Can you work these out from the model? Positions are in its coordinate system, mm. Face numbers are marked on the shaded views. Coordinates: 2 decimals unless noted, no trailing zeros. Loops run counter-clockwise (first coordinate to the right, second up) from the corner with the lowest first, then second, coordinate; pieces in that order, holes last.
```python
from build123d import *

# Parameters (mm, degrees)
F1_DEPTH  = 8
F3_DEPTH  = 50
F4_R      = 5
F5_DEPTH  = 9
F7_DEPTH  = 8
F9_DEPTH  = 25
F11_DEPTH = 65
F12_DEPTH = 1
F13_R     = 5
F14_R     = 2
F15_R     = 2


with BuildPart() as f1:
    # F0 (on Top) → F1 (new body)
    with BuildSketch(Plane.XY):
        Polygon((-15, 0), (0, 0), (10, 0), (10, 15), (10, 25), (5, 25), (5, 17), (-5, 17), (-13, 17), (-13, 25), (-20, 25), (-20, 0), align=None)
        with BuildLine():
            Line((10, 0), (0, 0))
            Line((0, 0), (-15, 0))
            ThreePointArc((-15, 0), (-4.7480671489, -26.7494728588), (0, -55))
            Line((0, -55), (10, -55))
            Line((10, -55), (10, 0))
        make_face()
        with BuildLine():
            ThreePointArc((16.1671913498, -8.6829612821), (13.2107261045, -4.2511845243), (10, 0))
            Line((10, 0), (10, -55))
            Line((10, -55), (30, -55))
            ThreePointArc((30, -55), (26.2150971911, -30.9062424985), (16.1671913498, -8.6829612821))
        make_face()
    extrude(amount=F1_DEPTH)

    # F2 (on face) → F3 (cut)
    with BuildSketch(Plane.YZ.offset(10)):
        with BuildLine():
            Line((22, 4), (24.5, 4))
            ThreePointArc((24.5, 4), (22, 6.5), (19.5, 4))
            Line((19.5, 4), (22, 4))
        make_face()
        with BuildLine():
            ThreePointArc((19.5, 4), (22, 1.5), (24.5, 4))
            Line((24.5, 4), (22, 4))
            Line((22, 4), (19.5, 4))
        make_face()
    extrude(amount=-F3_DEPTH, mode=Mode.SUBTRACT)

    # F4 (on face) → F5 (join)
    with BuildSketch(Plane(origin=(0, 0, 0), x_dir=(1, 0, 0), z_dir=(0, 0, -1))):
        with Locations((5, 0)):
            Circle(F4_R)
    extrude(amount=-F5_DEPTH)

    # F6 (on face) → F7 (join)
    with BuildSketch(Plane.XY.offset(9)):
        with BuildLine():
            ThreePointArc((1.05, 0), (5, -3.95), (8.95, 0))
            Line((8.95, 0), (1.05, 0))
        make_face()
        with BuildLine():
            Line((1.05, 0), (8.95, 0))
            ThreePointArc((8.95, 0), (5, 3.95), (1.05, 0))
        make_face()
    extrude(amount=F7_DEPTH)

    # F8 (on face) → F9 (cut)
    with BuildSketch(Plane.XY.offset(17)):
        with BuildLine():
            Line((2.5, 0), (7.5, 0))
            ThreePointArc((7.5, 0), (5, 2.5), (2.5, 0))
        make_face()
        with BuildLine():
            ThreePointArc((2.5, 0), (5, -2.5), (7.5, 0))
            Line((7.5, 0), (2.5, 0))
        make_face()
    extrude(amount=-F9_DEPTH, mode=Mode.SUBTRACT)

    # F10 (on face) → F11 (join)
    with BuildSketch(Plane(origin=(-20, 0, 0), x_dir=(0, -1, 0), z_dir=(-1, 0, 0))):
        with BuildLine():
            ThreePointArc((-4, 0), (-1.1715728753, 1.1715728753), (0, 4))
            ThreePointArc((0, 4), (-1.1715728753, 6.8284271247), (-4, 8))
            ThreePointArc((-4, 8), (-8, 4), (-4, 0))
        make_face()
    extrude(amount=F11_DEPTH)

    # F12 (add): faces of the model
    f12_faces = [f1.faces().sort_by_distance(p)[0] for p in [
        (-16.5, 25, 4),
        (7.5, 25, 4),
    ]]
    extrude(f12_faces, amount=F12_DEPTH)

    # F13
    f13_edges = [f1.edges().sort_by_distance(p)[0] for p in [
        (0, -55, 4),
    ]]
    fillet(f13_edges, radius=F13_R)

    # F14
    f14_edges = [f1.edges().sort_by_distance(p)[0] for p in [
        (30, -55, 4),
    ]]
    fillet(f14_edges, radius=F14_R)

    # F15
    f15_edges = [f1.edges().sort_by_distance(p)[0] for p in [
        (-16.5, 26, 8),
        (7.5, 26, 8),
        (7.5, 26, 0),
        (-16.5, 26, 0),
    ]]
    fillet(f15_edges, radius=F15_R)


solid = f1.part
```
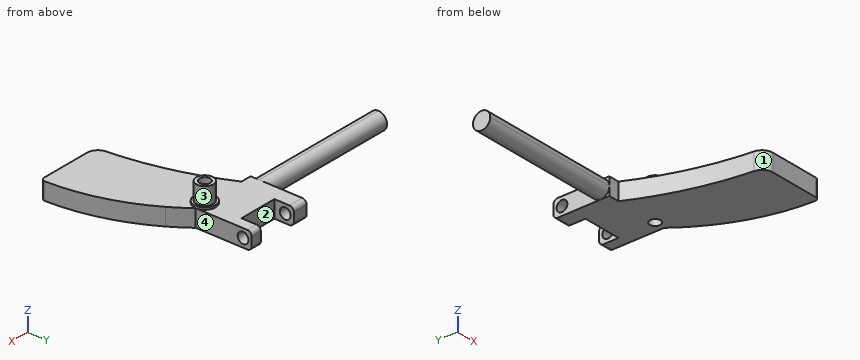
(1) I want a section at D-D on y = -45.5. Write out the boundary of the cut face in (x, z).
Check values:
outline: (-0.95, 0) - (29.3, 0) - (29.3, 8) - (-0.95, 8) - close
(2) I want a section at B-B on z = 11. Write out the boundary of the cut face in (x, y), then the cut area to 3 significant figures.
Check values:
outline: circle Ø7.9 at (5, 0); hole circle Ø5 at (5, 0)
area: 29.4 mm2
(3) I want a section at C-C on x = -55.5. Write out the boundary of the cut face in (y, z).
Check values:
outline: circle Ø8 at (4, 4)
(4) If we mould it in two halves opening along X, with no side actions, what happens to the marked faces 1, 2, 3 and 4? For each: released by +X, released by -X, zero draft, split by the parting line, or undercut.
Check values:
face 1: released by -X
face 2: undercut
face 3: split by the parting line
face 4: released by +X
(5) If I drill on probe 1 along Z at (x, y) = (-16.75, 22); probe 2 along X at (y, z) = (21, 1.5); probe 3 along Z at (x, y) = (18.5, -36.5), over which ranges is the centre line in solid material (lowest first)?
Check values:
probe 1: z = 0 to 1.5, 6.5 to 8
probe 2: x = -20 to -13, 5 to 10
probe 3: z = 0 to 8
(6) I want a section at A-A on y = 22. Write out the boundary of the cut face in (x, z), then the cut area to 3 significant figures.
Check values:
outline: (-20, 0) - (-13, 0) - (-13, 1.5) - (-20, 1.5) - close; (-20, 6.5) - (-13, 6.5) - (-13, 8) - (-20, 8) - close; (5, 0) - (10, 0) - (10, 1.5) - (5, 1.5) - close; (5, 6.5) - (10, 6.5) - (10, 8) - (5, 8) - close
area: 36.0 mm2
(7) I'm going to push flat-ended pins straight in: pin 1 (3 mm diameter, centred on y = 22, z = 4, fed in from +X); pin 2 (6.5 mm diameter, centred on y = 18.5, z = 4.5, fed in from +X); pin 3 (8 mm diameter, centred on y = -10, z = 10, fed in from -X); pin 4 (4 mm diameter, centred on y = 20, z = 3, fed in from -X). Where does each tip first touch, or does it pass through?
Check values:
pin 1: passes through
pin 2: stops at x = 10
pin 3: stops at x = -11.92
pin 4: stops at x = -20
